Work out the finished part from the listing and answer in its coordinate system (mm). A direction names the side the tool comes from. Coordinates: 2 decimals unless noted, no trailing zeros. Answer as a JSON object with one key per item and string values. Group by question number.
1) Find the intervals of material crossed by line 1 along X through (y, z) = (-0.5, -0.5); line 2 along X through (y, z) = (0.5, 0.25); line 3 along Z through (x, y) = (-1.5, -4), in increasing order.
2) The mould has two halves that part along X. Classify faces 3 (the face through (-3, 0, -0.9)), 4 (the face through (2.2, 0, 1)), 5 (the face through (-3, -1.5, 1)): released by +X, released by -X, zero draft, split by the parting line, or undercut.
3) Each of these flat-tipped pins is pushed along its axis until it touches: P1, Ø6, axis at x = -6, y = 5.5, coming from the -Z side; P2, Ø3, axis at x = 4.5, z = 2, coming from the +Y side; P3, Ø2, axis at y = -0.5, z = 2, coming from the -X side. Where does it stop, or does it pass through?
4) A tool of negligible diameter and unlimited length cuts with its end or side. For faces 1 (the face through (0, 0, 5.8)), 2 (the face through (3, 1.5, 1)), from which of +Z, -Z, +X, -X, +Y, -Y can it reach the whole face along a straight path? Write none if from no direction.
5) Section A-A (z = 0.25) is taken. Count the separate pieces of the cut face and the enclosed holes in it, plus the area to 3 significant figures.
from build123d import *

# Parameters (mm, degrees)
SKETCH003_W = 16
SKETCH003_H = 16
SKETCH004_W = 14
SKETCH004_H = 14
SKETCH_W    = 14.5
SKETCH_H    = 14.1
SKETCH005_W = 12.7
SKETCH005_H = 13.1
SKETCH006_W = 1
SKETCH006_H = 3
PAD_DEPTH   = 4
FILLET_R    = 2
FILLET001_R = 1
FILLET002_R = 0.5


with BuildPart() as part:
    # Sketch003 → AdditiveLoft section 0
    with BuildSketch(Plane.XY):
        Rectangle(SKETCH003_W, SKETCH003_H)
    # Sketch004 → AdditiveLoft section 1
    with BuildSketch(Plane.XY.offset(5.8)):
        Rectangle(SKETCH004_W, SKETCH004_H)
    loft()

    # Sketch (on Face1 of AdditiveLoft) → SubtractiveLoft section 0
    with BuildSketch(Plane(origin=(0, 0, 0), x_dir=(1, 0, 0), z_dir=(0, 0, -1))):
        Rectangle(SKETCH_W, SKETCH_H)
    # Sketch005 → SubtractiveLoft section 1
    with BuildSketch(Plane.XY.offset(3.1)):
        Rectangle(SKETCH005_W, SKETCH005_H)
    loft(mode=Mode.SUBTRACT)

    # Sketch006 (on Face11 of SubtractiveLoft) → Pad (new body)
    with BuildSketch(Plane(origin=(0, 0, 3.1), x_dir=(1, 0, 0), z_dir=(0, 0, -1))):
        with Locations((-2.7, 0)):
            Rectangle(SKETCH006_W, SKETCH006_H)
    pad = extrude(amount=PAD_DEPTH)

    # Mirrored: Pad across Sketch006 V_Axis
    add(pad.mirror(Plane(origin=(0, 0, 3.1), x_dir=(0, 0, -1), z_dir=(1, 0, 0))))

    # Fillet
    fillet_edges = [part.edges().sort_by_distance(p)[0] for p in [
        (-7.5, -7.5, 2.9),
        (-7.5, 7.5, 2.9),
        (7.5, 7.5, 2.9),
        (7.5, -7.5, 2.9),
    ]]
    fillet(fillet_edges, radius=FILLET_R)

    # Fillet001
    fillet001_edges = [part.edges().sort_by_distance(p)[0] for p in [
        (-6.8, -6.8, 1.55),
        (-6.8, 6.8, 1.55),
        (6.8, -6.8, 1.55),
        (6.8, 6.8, 1.55),
    ]]
    fillet(fillet001_edges, radius=FILLET001_R)

    # Fillet002
    fillet002_edges = [part.edges().sort_by_distance(p)[0] for p in [
        (-2.2, 0, 3.1),
        (-2.7, -1.5, 3.1),
        (2.7, -1.5, 3.1),
        (3.2, 0, 3.1),
        (2.7, 1.5, 3.1),
        (-2.7, 1.5, 3.1),
        (2.2, 0, 3.1),
        (-3.2, 0, 3.1),
    ]]
    fillet(fillet002_edges, radius=FILLET002_R)


solid = part.part
Report:
{
 "1": {"line 1": "x = -3.2 to -2.2, 2.2 to 3.2", "line 2": "x = -7.96 to -7.18, -3.2 to -2.2, 2.2 to 3.2, 7.18 to 7.96", "line 3": "z = 3.1 to 5.8"},
 "2": {"face 3": "zero draft", "face 4": "undercut", "face 5": "undercut"},
 "3": {"P1": "stops at z = 0", "P2": "stops at y = 7.91", "P3": "stops at x = -7.83"},
 "4": {"face 1": "+Z, +X, -X, +Y, -Y", "face 2": "-Z"},
 "5": {"separate pieces": "3", "enclosed holes": "1", "area": "55.5 mm²"}
}
